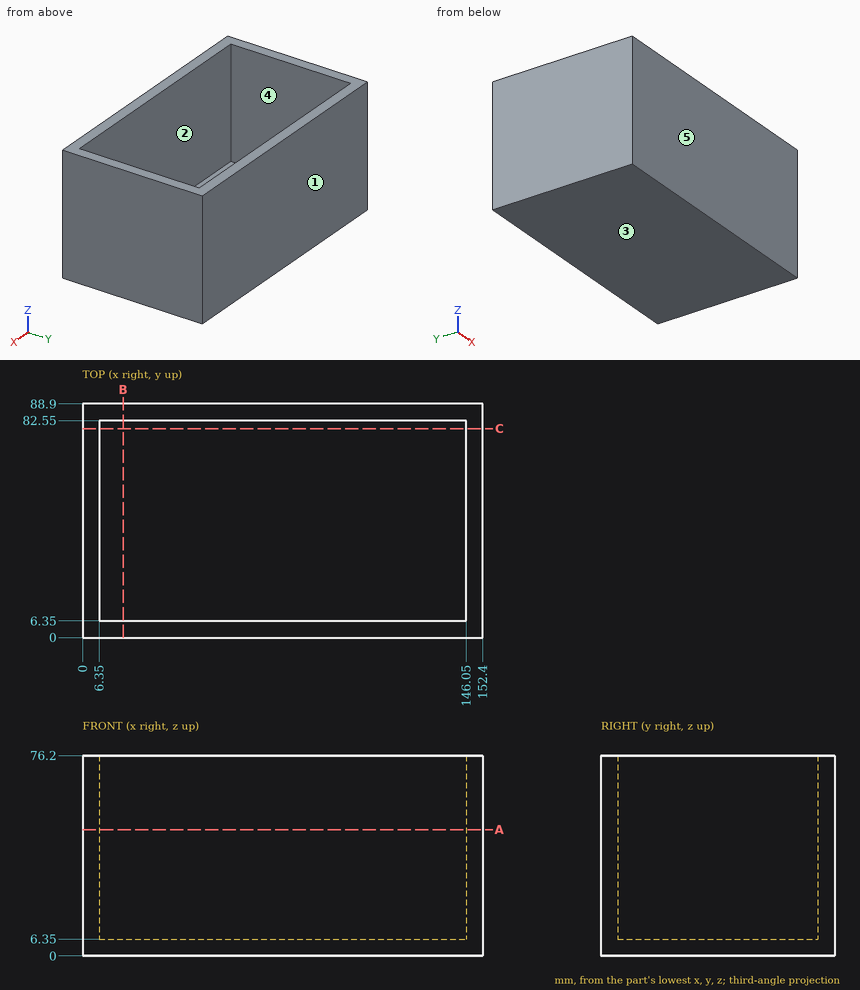
Geometry check sheet. Reference: drawing and pictorial views, mm from the part's lowest x, y, z. A direction names the side the tool comes from. Give positions to 0.01 mm unless a question says otherwise; leave off trailing zeros. Write each loop counter-clockwise with the first axis right and the second up, starting at its lowest first coordinate (ties: lowest second). Pieces come first, ordered by that corner, then holes. Notation, with made-up numbers: (30, 0) - (47, 0) arc R12 cw to (47, 14) - close; hole circle Ø3 at (35.25, 35). An arc over 180 degrees is marked (long way). Put each result on its own line as item: value.
Q1. Section check A-A on z = 48. Record the cut outline in (x, y).
Result:
outline: (0, 0) - (152.4, 0) - (152.4, 88.9) - (0, 88.9) - close; hole (6.35, 6.35) - (146.05, 6.35) - (146.05, 82.55) - (6.35, 82.55) - close
Q2. Mould release check, pull along Y, two halves, no side actions. Record for the marked faces 3, 4 and 5: released by +Y, released by -Y, zero draft, split by the parting line, or undercut.
Result:
face 3: zero draft
face 4: undercut
face 5: released by -Y
Q3. Depth check by flat-ended pin: P1, Ø5, axis at x = 49.5, y = 64.5, coming from the +Z side. Enter the tip coordinate at first touch or a pass-through.
Result:
P1: z = 6.35
Q4. Section check C-C on y = 79.5. Record the cut outline in (x, z).
Result:
outline: (0, 0) - (152.4, 0) - (152.4, 76.2) - (146.05, 76.2) - (146.05, 6.35) - (6.35, 6.35) - (6.35, 76.2) - (0, 76.2) - close
Q5. Scan lines: probe 1 along X at (y, z) = (74, 48.5); probe 2 along Y at (x, z) = (114, 41); probe 3 along Z at (x, y) = (54, 69). Record each from-to range of solid material in increasing order. Write a range as from..to.
Result:
probe 1: 0..6.35, 146.05..152.4
probe 2: 0..6.35, 82.55..88.9
probe 3: 0..6.35
Q6. Set-up check for the marked faces 1 and 2: record each of +Z, -Z, +X, -X, +Y, -Y from which the full face is reachable in a straight line by a thin tool's end or side.
Result:
face 1: +Z, -Z, +X, -X, +Y
face 2: +Z
Q7. Section check B-B on x = 15.5. Record the cut outline in (y, z).
Result:
outline: (0, 0) - (88.9, 0) - (88.9, 76.2) - (82.55, 76.2) - (82.55, 6.35) - (6.35, 6.35) - (6.35, 76.2) - (0, 76.2) - close
